CAD build for the part. Positions are in the model's coordinates, mm. Round coordinates to 2 decimals unless told otherwise and drop trailing zeros. Order: outer loops, then holes, each group sorted by start corner. A loop starts at its lowest first (then second) coordinate and runs counter-clockwise, first axis right, second up. Notation, with made-up numbers: (61.25, 42) - (69.25, 42) arc R33 cw to (69.25, 80) - close; hole circle Ø9 at (73.25, 25). An arc over 180 degrees is marked (long way). Write item = value, one per line.
Autodesk Inventor part; units mm, degrees
ref_plane "YZ Plane" through (0, 0, 0) normal (1, 0, 0) x (0, 1, 0)
ref_plane "XZ Plane" through (0, 0, 0) normal (0, 1, 0) x (-1, 0, 0)
ref_plane "XY Plane" through (0, 0, 0) normal (0, 0, 1) x (1, 0, 0)
sketch "Sketch1" plane through (0, 0, 0) normal (0, 1, 0) x (-1, 0, 0)
  line L0 (49, 0) -> (0, 0)
  line L1 (0, 0) -> (0, -38)
  line L2 (0, -38) -> (49, -38)
  line L3 (49, -38) -> (49, 0)
  dimension "d0" = 38
  dimension "d1" = 49
extrude "Extrusion1" add sketch "Sketch1" along normal blind 1.6
sketch "Sketch2" plane through (0, 1.6, 0) normal (0, 1, 0) x (1, 0, 0)
  line L0 (-49, 38) -> (-49, 0) construction
  line L1 (-49, 19) -> (0, 19) construction
  line L2 (0, 0) -> (0, 38) construction
  line L3 (0, 38) -> (-49, 38)
  point P0 (-13.65, 3)
  point P1 (-13.65, 35)
  point P2 (-46, 35)
  point P3 (-46, 3)
  dimension "d5" = 32.35
  dimension "d6" = 3
  dimension "d14" = 3
hole "Hole1" at (-13.65, 1.6, -3) at (-13.65, 1.6, -35) at (-46, 1.6, -35) at (-46, 1.6, -3) direction (0, -1, 0) diameter 4.305 end through all
properties part number "_Reference_PCB"
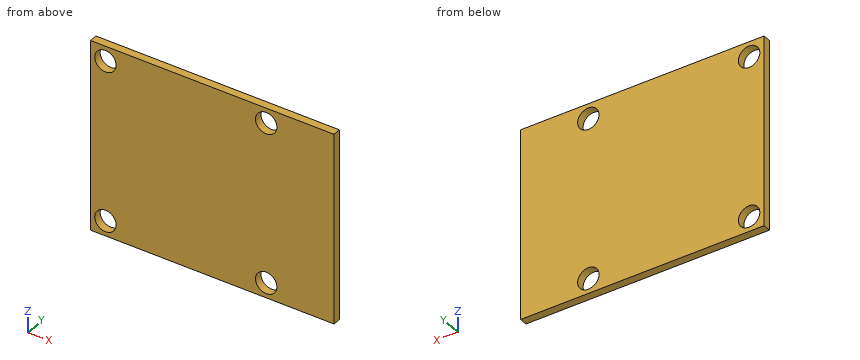
(1) Drop a flat-ended pin along its axis: pin 1 (4 mm diameter, centred on x = -46, z = -35, fed in from -Y). Give the stop position or say it passes through.
Solved:
pin_1 = through
(2) Band-saw the part on A-A on x = -46. List the corners of the cut face in (y, z).
Solved:
outline = (0, -38) - (1.6, -38) - (1.6, -37.15) - (0, -37.15) - close; (0, -32.85) - (1.6, -32.85) - (1.6, -5.15) - (0, -5.15) - close; (0, -0.85) - (1.6, -0.85) - (1.6, 0) - (0, 0) - close
(3) Band-saw the part on C-C on z = -3. List the corners of the cut face in (x, y), plus the area to 3 significant figures.
Solved:
outline = (-49, 0) - (-48.15, 0) - (-48.15, 1.6) - (-49, 1.6) - close; (-43.85, 0) - (-15.8, 0) - (-15.8, 1.6) - (-43.85, 1.6) - close; (-11.5, 0) - (0, 0) - (0, 1.6) - (-11.5, 1.6) - close
area = 64.6 mm²
(4) Band-saw the part on B-B on y = 1.1. Count the separate pieces of the cut face and the enclosed holes in it, plus the area to 3 significant figures.
Solved:
separate_pieces = 1
enclosed_holes = 4
area = 1,800 mm²
(5) Probe line 1 along X through (y, z) = (1.3, -3); line 2 along Z through (x, y) = (-13.65, 1); line 3 along Z through (x, y) = (-45.5, 0.95). List the from-to ranges inside material, lowest first.
Solved:
line_1 = -49 to -48.15, -43.85 to -15.8, -11.5 to 0
line_2 = -38 to -37.15, -32.85 to -5.15, -0.85 to 0
line_3 = -38 to -37.09, -32.91 to -5.09, -0.91 to 0
